Design review of the part built by this model. Coordinates are the model's own, in mm. A direction names the side the tool comes from. Give positions to 0.01 mm unless a question says otherwise; leave off trailing zeros. Loops run counter-clockwise (first coordinate to the right, second up) from the corner with the lowest first, then second, coordinate; pieces in that order, holes last. Notation, with made-up numbers: (80.5, 83.25) -> (115.5, 83.25) arc R20 ccw to (115.5, 90.25) -> close; hole circle Ø6 at (84.5, 28.5). An arc over 180 degrees is marked (long way). Answer as CSV lines item,"result".
from build123d import *

# Parameters (mm, degrees)
SKETCH1_W            = 105.1814
SKETCH1_H            = 68.320954018
BOSS_EXTRUDE1_DEPTH  = 4.5085
SKETCH2_W            = 105.1814
SKETCH2_H            = 15.933454036
CUT_EXTRUDE1_DEPTH   = 10.795
SKETCH3_W            = 6.35
SKETCH3_H            = 12.7
BOSS_EXTRUDE2_DEPTH  = 4.5085
CUT_EXTRUDE2_DEPTH   = 4.7625
LPATTERN1_COUNT      = 3
LPATTERN1_PITCH      = 39.916133528
CUT_EXTRUDE3_DEPTH   = 4.7625
FILLET2_R            = 1.905
MIRROR3_COPY_1_DEPTH = 4.7625
MIRROR3_COPY_2_DEPTH = 4.7625
MIRROR3_COPY_3_DEPTH = 4.7625
FILLET3_R            = 1.905
SKETCH6_W            = 3.302
SKETCH6_H            = 6.35
CUT_EXTRUDE4_DEPTH   = 6.35


with BuildPart() as part:
    # Sketch1 → Boss-Extrude1 (new body)
    with BuildSketch(Plane.XY):
        Rectangle(SKETCH1_W, SKETCH1_H)
    extrude(amount=BOSS_EXTRUDE1_DEPTH)

    # Sketch2 → Cut-Extrude1 (cut)
    with BuildSketch(Plane.XY.offset(4.5085)):
        with Locations((0, 26.193749991)):
            Rectangle(SKETCH2_W, SKETCH2_H)
    extrude(amount=-CUT_EXTRUDE1_DEPTH, mode=Mode.SUBTRACT)

    # Sketch3 → Boss-Extrude2 (add)
    with BuildSketch(Plane.XY.offset(4.5085)):
        with Locations((-55.7657, -27.810477009)):
            Rectangle(SKETCH3_W, SKETCH3_H)
        with Locations((-55.7657, 11.877022991)):
            Rectangle(SKETCH3_W, SKETCH3_H)
    boss_extrude2 = extrude(amount=-BOSS_EXTRUDE2_DEPTH)

    # Mirror1: Boss-Extrude2 across plane
    add(boss_extrude2.mirror(Plane(origin=(0, 0, 0), x_dir=(0, 0, 1), z_dir=(1, 0, 0))))

    # Sketch4 → Cut-Extrude2 (cut)
    with BuildSketch(Plane(origin=(0, 0, 0), x_dir=(-1, 0, 0), z_dir=(0, 0, -1))):
        Polygon((-49.4157, 15.052022991), (-30.3657, 15.052022991), (-39.8907, -3.997977009), align=None)
    cut_extrude2 = extrude(amount=-CUT_EXTRUDE2_DEPTH, mode=Mode.SUBTRACT)

    # LPattern1: Cut-Extrude2 ×3
    with Locations(*[(-i * LPATTERN1_PITCH, 0, 0) for i in range(1, LPATTERN1_COUNT)]):
        add(cut_extrude2, mode=Mode.SUBTRACT)

    # Sketch5 → Cut-Extrude3 (cut)
    with BuildSketch(Plane(origin=(0, 0, 0), x_dir=(-1, 0, 0), z_dir=(0, 0, -1))):
        Polygon((-27.1907, 15.052022991), (-12.674566472, 15.052022991), (-3.149566472, -3.997977009), (-36.7157, -3.997977009), align=None)
    cut_extrude3 = extrude(amount=-CUT_EXTRUDE3_DEPTH, mode=Mode.SUBTRACT)

    # Mirror2: Cut-Extrude3 across plane
    add(cut_extrude3.mirror(Plane(origin=(0, 0, 0), x_dir=(0, 0, 1), z_dir=(1, 0, 0))), mode=Mode.SUBTRACT)

    # Fillet2
    fillet2_edges = [part.edges().sort_by_distance(p)[0] for p in [
        (-0.025433528, -3.997977009, 2.25425),
        (9.499566472, 15.052022991, 2.25425),
        (-9.550433528, 15.052022991, 2.25425),
        (-30.416567056, 15.052022991, 2.25425),
        (-39.941567056, -3.997977009, 2.25425),
        (-49.466567056, 15.052022991, 2.25425),
        (39.8907, -3.997977009, 2.25425),
        (49.4157, 15.052022991, 2.25425),
        (30.3657, 15.052022991, 2.25425),
    ]]
    fillet(fillet2_edges, radius=FILLET2_R)

    # Mirror3: Cut-Extrude2, Cut-Extrude3 across plane
    add(cut_extrude2.mirror(Plane.ZX.offset(-7.966727018)), mode=Mode.SUBTRACT)
    add(cut_extrude3.mirror(Plane.ZX.offset(-7.966727018)), mode=Mode.SUBTRACT)

    # Mirror3 copy 1 sketch → Mirror3 copy 1 (cut)
    with BuildSketch(Plane(origin=(-39.916133528, -15.933454036, 0), x_dir=(-1, 0, 0), z_dir=(0, 0, -1))):
        Polygon((-49.4157, -15.052022991), (-30.3657, -15.052022991), (-39.8907, 3.997977009), align=None)
    extrude(amount=-MIRROR3_COPY_1_DEPTH, mode=Mode.SUBTRACT)

    # Mirror3 copy 2 sketch → Mirror3 copy 2 (cut)
    with BuildSketch(Plane(origin=(-79.832267056, -15.933454036, 0), x_dir=(-1, 0, 0), z_dir=(0, 0, -1))):
        Polygon((-49.4157, -15.052022991), (-30.3657, -15.052022991), (-39.8907, 3.997977009), align=None)
    extrude(amount=-MIRROR3_COPY_2_DEPTH, mode=Mode.SUBTRACT)

    # Mirror3 copy 3 sketch → Mirror3 copy 3 (cut)
    with BuildSketch(Plane(origin=(0, -15.933454036, 0), x_dir=(1, 0, 0), z_dir=(0, 0, -1))):
        Polygon((-27.1907, 15.052022991), (-12.674566472, 15.052022991), (-3.149566472, -3.997977009), (-36.7157, -3.997977009), align=None)
    extrude(amount=-MIRROR3_COPY_3_DEPTH, mode=Mode.SUBTRACT)

    # Fillet3
    fillet3_edges = [part.edges().sort_by_distance(p)[0] for p in [
        (36.7157, -3.997977009, 2.25425),
        (27.1907, 15.052022991, 2.25425),
        (12.674566472, 15.052022991, 2.25425),
        (3.149566472, -3.997977009, 2.25425),
        (-27.1907, 15.052022991, 2.25425),
        (-36.7157, -3.997977009, 2.25425),
        (-3.149566472, -3.997977009, 2.25425),
        (-12.674566472, 15.052022991, 2.25425),
        (49.4157, -30.985477027, 2.25425),
        (39.8907, -11.935477027, 2.25425),
        (30.3657, -30.985477027, 2.25425),
        (9.499566472, -30.985477027, 2.25425),
        (-0.025433528, -11.935477027, 2.25425),
        (-9.550433528, -30.985477027, 2.25425),
        (-30.416567056, -30.985477027, 2.25425),
        (-39.941567056, -11.935477027, 2.25425),
        (-49.466567056, -30.985477027, 2.25425),
        (-36.7157, -11.935477027, 2.25425),
        (-27.1907, -30.985477027, 2.25425),
        (-12.674566472, -30.985477027, 2.25425),
        (-3.149566472, -11.935477027, 2.25425),
        (27.1907, -30.985477027, 2.25425),
        (36.7157, -11.935477027, 2.25425),
        (3.149566472, -11.935477027, 2.25425),
        (12.674566472, -30.985477027, 2.25425),
    ]]
    fillet(fillet3_edges, radius=FILLET3_R)

    # Sketch6 → Cut-Extrude4 (cut)
    with BuildSketch(Plane(origin=(0, 0, 0), x_dir=(-1, 0, 0), z_dir=(0, 0, -1))):
        with Locations((-54.2417, 8.702022991)):
            Rectangle(SKETCH6_W, SKETCH6_H)
        with Locations((54.2417, 8.702022991)):
            Rectangle(SKETCH6_W, SKETCH6_H)
        with Locations((-54.2417, -30.985477009)):
            Rectangle(SKETCH6_W, SKETCH6_H)
        with Locations((54.2417, -30.985477009)):
            Rectangle(SKETCH6_W, SKETCH6_H)
    extrude(amount=-CUT_EXTRUDE4_DEPTH, mode=Mode.SUBTRACT)


solid = part.part
Q1. Clearance check with a flat-ended pin moving along its axis: pin 1 Ø1 at (x, z) = (-54, 2) entering from -Y. State where the tip first meets the part, or that it passes through.
Filled sheet:
pin 1,"stops at y = -27.81"
Q2. We need section B-B, the plane y = -16.5. State the section outline as (x, z) points, and give its area (3 significant figures).
Filled sheet:
outline,"(-52.59, 0) -> (-42.22, 0) -> (-42.22, 4.51) -> (-52.59, 4.51) -> close; (-37.66, 0) -> (-34.43, 0) -> (-34.43, 4.51) -> (-37.66, 4.51) -> close; (-5.43, 0) -> (-2.31, 0) -> (-2.31, 4.51) -> (-5.43, 4.51) -> close; (2.26, 0) -> (5.43, 0) -> (5.43, 4.51) -> (2.26, 4.51) -> close; (34.43, 0) -> (37.61, 0) -> (37.61, 4.51) -> (34.43, 4.51) -> close; (42.17, 0) -> (52.59, 0) -> (52.59, 4.51) -> (42.17, 4.51) -> close"
area,"151 mm^2"
Q3. We need section D-D, the plane x = 10.5. State the section outline as (y, z) points.
Filled sheet:
outline,"(-34.16, 0) -> (-26.64, 0) -> (-26.64, 4.51) -> (-34.16, 4.51) -> close; (-11.94, 0) -> (-4, 0) -> (-4, 4.51) -> (-11.94, 4.51) -> close; (10.7, 0) -> (18.23, 0) -> (18.23, 4.51) -> (10.7, 4.51) -> close"
Q4. For faces 3 (the flat face through (-12, -8, 4.508)), 4 (the flat face through (40, 15.052, 2)), 5 (the flat face through (-52.591, -31, 2)), list the 3-axis set-ups (+Z, -Z, +X, -X, +Y, -Y) from which the entire face can be reached by the end or side of a thin tool; tool diameter is ignored.
Filled sheet:
face 3,"+Z, +X, -X, +Y, -Y"
face 4,"+Z, -Z"
face 5,"+Z, -Z, -Y"
Q5. To check wall thickness, follow probe 1 along Y at (x, z) = (26, 3.7); probe 2 along X at (y, z) = (-13, 2.15); probe 3 along X at (y, z) = (14, 2.45). State the ranges of each line that lie inside material, in increasing order. Write a range as from..to.
Filled sheet:
probe 1,"y = -34.16..-30.99, -11.94..-4, 15.05..18.23"
probe 2,"x = -52.59..-35.34, -4.52..4.52, 35.34..52.59"
probe 3,"x = -58.94..-48.09, -31.8..-27.72, -12.15..-8.17, 8.12..12.15, 27.72..31.74, 48.04..58.94"
Q6. We need section A-A, the plane x = -23. State the section outline as (y, z) points, and give its area (3 significant figures).
Filled sheet:
outline,"(-34.16, 0) -> (-30.99, 0) -> (-30.99, 4.51) -> (-34.16, 4.51) -> close; (-11.94, 0) -> (-4, 0) -> (-4, 4.51) -> (-11.94, 4.51) -> close; (15.05, 0) -> (18.23, 0) -> (18.23, 4.51) -> (15.05, 4.51) -> close"
area,"64.4 mm^2"
Q7. The part is to be moulded in two halves that separate along X. For faces 1 (the cylindrical face through (39.92, -14.29, 2.29)), 2 (the flat face through (-1, 18.227, 2)), say which applies: pulls with the +X half, pulls with the -X half, needs draft (parallel to the pull), parting line crosses it, or undercut.
Filled sheet:
face 1,"undercut"
face 2,"needs draft"
Q8. We need section C-C, the plane z = 3.3. State how many separate pieces and enclosed holes the cut face has, and give its area (3 significant figures).
Filled sheet:
separate pieces,"1"
enclosed holes,"10"
area,"2,890 mm^2"
